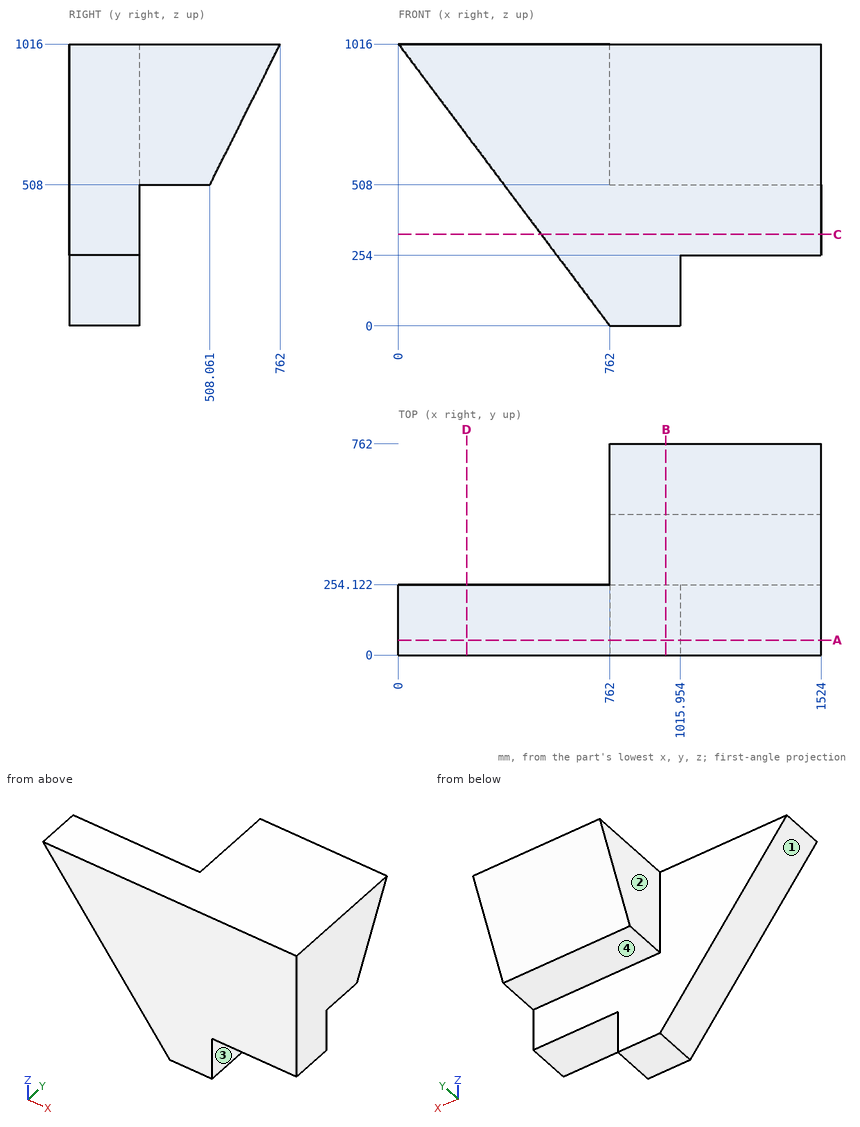
Study the drawing (mm; zero at the part's minimum x, y, z) and answer. A direction names the side the tool comes from. Round coordinates to 2 decimals unless told otherwise and drop trailing zeros. Order: outer loops, then holes, each group sorted by start corner. A loop starts at its lowest first (then second) coordinate and runs counter-clockwise, first axis right, second up. Notation, with made-up numbers: (80, 30.5) -> (121, 30.5) arc R26 cw to (121, 56.5) -> close; hole circle Ø3 at (-1.75, 37). An arc over 180 degrees is marked (long way). Answer as CSV lines item,"result". Start each with the question number.
(1) The part is cut by section D-D (x = 246). Determine the outline of the cut face in (y, z), then the cut area to 3 significant figures.
(2) Flat-ended cylindrical pins translate along their axes: pin 1 Ø8 at (x, z) = (503, 484.5) entering from +Y; pin 2 Ø6 at (y, z) = (608.5, 772.5) entering from -X; pin 3 Ø4 at (x, z) = (480, 601) entering from -Y. Find the tip coordinate at first contact, or state that the pin passes through.
(3) The part is cut by section B-B (x = 965). Determine the outline of the cut face in (y, z), then the cut area to 3 significant figures.
(4) The part is cut by section A-A (y = 54). Determine the outline of the cut face in (x, z), then the cut area to 3 significant figures.
(5) Find the intervals of material crossed by probe 1 along Y at (x, z) = (547, 612.5); probe 2 along X at (y, z) = (314, 789); probe 3 along Z at (x, y) = (1255, 158), in increasing order. Write a range as from..to.
(6) The part is cut by section C-C (z = 330). Determine the outline of the cut face in (x, y).
(7) A tool of negligible diameter and unlimited length cuts with its end or side. For the marked faces 1, 2, 3 and 4, from which of +Z, -Z, +X, -X, +Y, -Y can it reach the whole face along a straight path? Write none if from no direction.
Evaluation:
1,outline,"(0, 688) -> (254.12, 688) -> (254.12, 1016) -> (0, 1016) -> close"
1,area,"83,400 mm²"
2,pin 1,"y = 254.12"
2,pin 2,"x = 762"
2,pin 3,"y = 0"
3,outline,"(0, 0) -> (254.12, 0) -> (254.12, 508) -> (508.06, 508) -> (762, 1016) -> (0, 1016) -> close"
3,area,"452,000 mm²"
4,outline,"(0, 1016) -> (762, 0) -> (1015.95, 0) -> (1015.95, 254) -> (1524, 254) -> (1524, 1016) -> close"
4,area,"1,030,000 mm²"
5,probe 1,"0..254.12"
5,probe 2,"762..1524"
5,probe 3,"254..1016"
6,outline,"(514.5, 0) -> (1524, 0) -> (1524, 254.12) -> (514.5, 254.12) -> close"
7,face 1,"-Z, -X, +Y, -Y"
7,face 2,"+Z, -Z, -X, +Y"
7,face 3,"-Z, +X, +Y, -Y"
7,face 4,"-Z, +X, -X, +Y"
